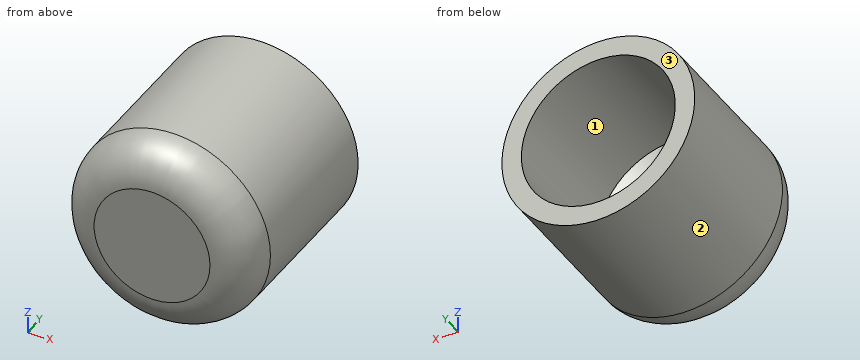
from build123d import *

# Parameters (mm, degrees)
F0_R     = 63.6455484586
F1_DEPTH = 127
F2_R     = 25.4
F4_D     = 101.6
F4_DEPTH = 88.9
F4_TIP   = 30.5237194466


with BuildPart() as f1:
    # F0 (on Front) → F1 (new body)
    with BuildSketch(Plane.XZ):
        Circle(F0_R)
    extrude(amount=F1_DEPTH)

    # F2
    f2_edges = [f1.edges().sort_by_distance(p)[0] for p in [
        (-63.645548, -127, 0),
    ]]
    fillet(f2_edges, radius=F2_R)

    # F4
    with Locations(Plane(origin=(0, 0, 0), x_dir=(-1, 0, 0), z_dir=(0, 1, 0))):
        with Locations((0, 0)):
            Hole(F4_D / 2, depth=F4_DEPTH)
            with Locations((0, 0, -(F4_DEPTH + F4_TIP / 2))):  # 118° drill point
                Cone(0, F4_D / 2, F4_TIP, mode=Mode.SUBTRACT)


solid = f1.part
The model under review builds one solid part; all positions refer to its coordinate system, in mm. Face numbers are marked on the shaded views. Give positions to 0.01 mm unless a question says otherwise; leave off trailing zeros. Loops run counter-clockwise (first coordinate to the right, second up) from the corner with the lowest first, then second, coordinate; pieces in that order, holes last. Notation, with made-up numbers: (72.5, -19.75) -> (78.5, -19.75) arc R32 ccw to (78.5, 12.25) -> close; hole circle Ø3 at (-7, -37.75). An arc over 180 degrees is marked (long way). Put each result on its own line as item: value. Start each with the question number.
1. Wall thickness on probe 1 along Z at (x, y) = (0, -28); probe 2 along Z at (x, y) = (14.5, -53); probe 3 along X at (y, z) = (-37.5, 43.5): over which ranges is each line inside the solid? List them lowest first.
2. We need section B-B on y = -92. State the section outline as (x, z) points, then the cut area to 3 significant figures.
3. We need section A-A on y = -26.5. State the section outline as (x, z) points.
4. Mouldability with a two-part tool opening along X and no side actions: class the marked faces 1, 2 and 3 as released by +X, released by -X, zero draft, split by the parting line, or undercut.
5. Clearance check with flat-ended pins moving along their axes: P1, Ø1.5, axis at x = 22.5, y = -111.5, coming from the -Z side; P2, Ø12, axis at x = -23, y = -13, coming from the +Z side; P3, Ø5, axis at y = -33, z = -40.5, coming from the +X side. State where each tip first meets the part, or that it passes through.
Determined:
1. probe 1: -63.65 to -50.8, 50.8 to 63.65
1. probe 2: -61.97 to -48.69, 48.69 to 61.97
1. probe 3: -46.46 to -26.24, 26.24 to 46.46
2. outline: circle Ø127.29 at (0, 0); hole circle Ø91.28 at (0, 0)
2. area: 6,180 mm^2
3. outline: circle Ø127.29 at (0, 0); hole circle Ø101.6 at (0, 0)
4. face 1: undercut
4. face 2: split by the parting line
4. face 3: zero draft
5. P1: z = -57.82
5. P2: z = 61.33
5. P3: x = 51.06
